Job drawing, mm, ordinate dimensions from the low corner. One solid piece. A direction names the side the tool comes from. Give positions to 0.01 mm unless a question says otherwise; leave off trailing zeros. Loops run counter-clockwise (first coordinate to the right, second up) from the corner with the lowest first, then second, coordinate; pieces in that order, holes last. Notation, with made-up numbers: (70.25, 85.5) -> (86.25, 85.5) arc R19 ccw to (86.25, 114.5) -> close; hole circle Ø10 at (13.25, 34.5). An arc over 180 degrees is marked (long way). Answer as a JSON object with one key per item and string values. Group by question number.
Q1. Wall check: probe 1 along X at (y, z) = (1.1, 3.5) (1 decimal); probe 2 along Y at (x, z) = (1, 2.75); probe 3 along Z at (x, y) = (5, 3.6). Give the ranges that are in metal, low to high. Write a range as from..to.
Q2. Band-saw the part on C-C, the plane x = 2.5. Write the cut outline in (y, z), plus the area to 3 significant figures.
Q3. Band-saw the part on D-D, the plane x = 6.75. Write the cut outline in (y, z).
Q4. Drop flat-ended pins along their axis: pin 1 (0.6 mm diameter, centred on x = 5, y = 4, fed in from -Z); pin 2 (2.5 mm diameter, centred on x = 4, z = 3.5, fed in from +Y); pin 3 (1 mm diameter, centred on y = 3.5, z = 4.5, fed in from +X). Give the stop position or say it passes through.
Q5. Tool access for the marked faces 4 and 5: list every direction of +Z, -Z, +X, -X, +Y, -Y with a clear straight run to the whole face (end or side of a thin tool).
Q6. Two-plate mould, pull along X, no slides. Class the marked faces 1, 2 and 3: pulls with the +X half, pulls with the -X half, needs draft (parallel to the pull), parting line crosses it, or undercut.
Q7. Band-saw the part on B-B, the plane z = 6.5. Write the cut outline in (x, y) (3 decimals).
Q8. Band-saw the part on A-A, the plane y = 1. Write the cut outline in (x, z) (3 decimals).
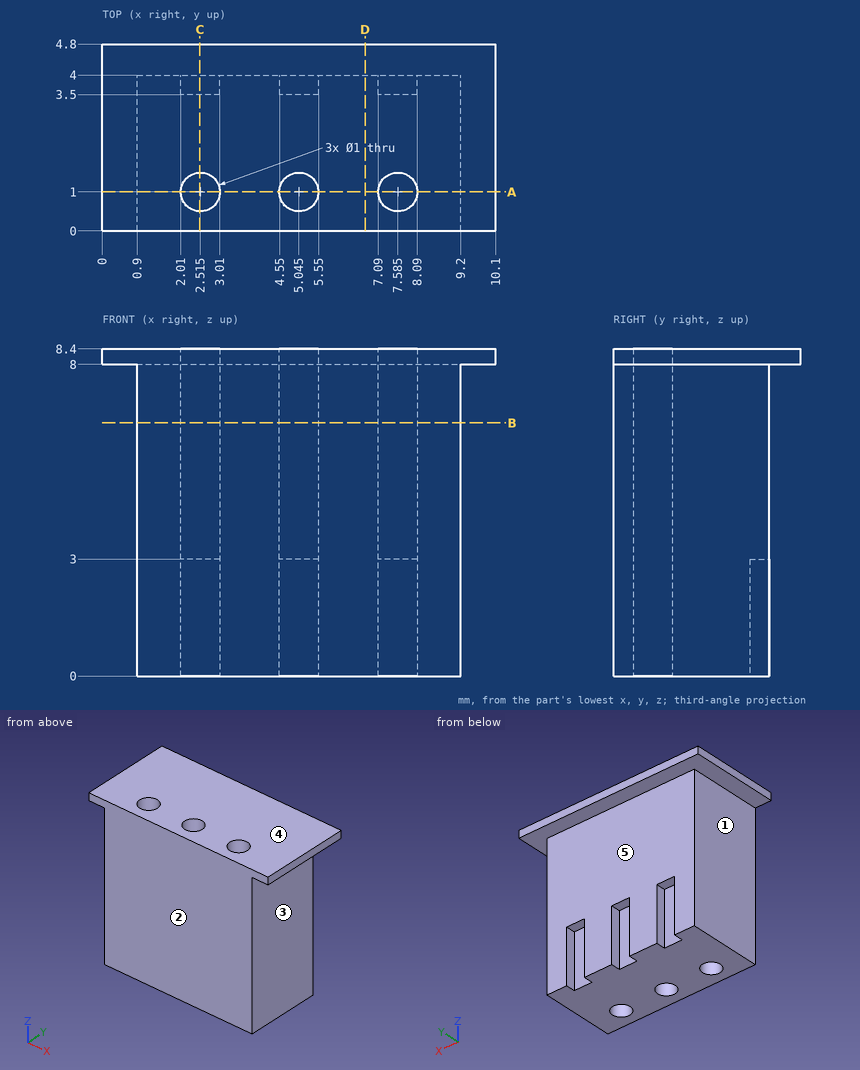
Worked answers:
{
 "1": {"probe 1": "0.9..2, 3..4.6, 5.5..7.1, 8.1..9.2", "probe 2": "0..4", "probe 3": "3..8.4"},
 "2": {"outline": "(0, 0) -> (0.5, 0) -> (0.5, 8.4) -> (0, 8.4) -> close; (1.5, 0) -> (3.5, 0) -> (3.5, 3) -> (4, 3) -> (4, 8) -> (4.8, 8) -> (4.8, 8.4) -> (1.5, 8.4) -> close", "area": "24.0 mm2"},
 "3": {"outline": "(0, 0) -> (4, 0) -> (4, 8) -> (4.8, 8) -> (4.8, 8.4) -> (0, 8.4) -> close"},
 "4": {"pin 1": "z = 3", "pin 2": "y = 4", "pin 3": "x = 9.2"},
 "5": {"face 4": "+Z, +X, -X, +Y, -Y", "face 5": "-Z, +X, -X, +Y"},
 "6": {"face 1": "pulls with the -X half", "face 2": "needs draft", "face 3": "pulls with the +X half"},
 "7": {"outline": "(0.9, 0) -> (9.2, 0) -> (9.2, 4) -> (0.9, 4) -> close; hole circle Ø1 at (2.515, 1); hole circle Ø1 at (5.045, 1); hole circle Ø1 at (7.585, 1)"},
 "8": {"outline": "(0, 8) -> (0.9, 8) -> (0.9, 0) -> (2.015, 0) -> (2.015, 8.4) -> (0, 8.4) -> close; (3.015, 0) -> (4.545, 0) -> (4.545, 8.4) -> (3.015, 8.4) -> close; (5.545, 0) -> (7.085, 0) -> (7.085, 8.4) -> (5.545, 8.4) -> close; (8.085, 0) -> (9.2, 0) -> (9.2, 8) -> (10.1, 8) -> (10.1, 8.4) -> (8.085, 8.4) -> close"}
}
